Answer from the drawing. Dimensions are ordinates in mm from the lowest x, y and z of the part. A direction names the side the tool comes from. Round coordinates to 2 decimals unless told otherwise and drop trailing zeros. Loops run counter-clockwise (first coordinate to the right, second up) from the corner with the lowest first, then second, coordinate; pieces in that order, holes last. Notation, with made-up numbers: M 0,53 L 34,53 A23 ccw 34,70 Z; hole C 41.25,-29.5 d8. An arc over 180 degrees is marked long. Answer as CSV lines item,"result".
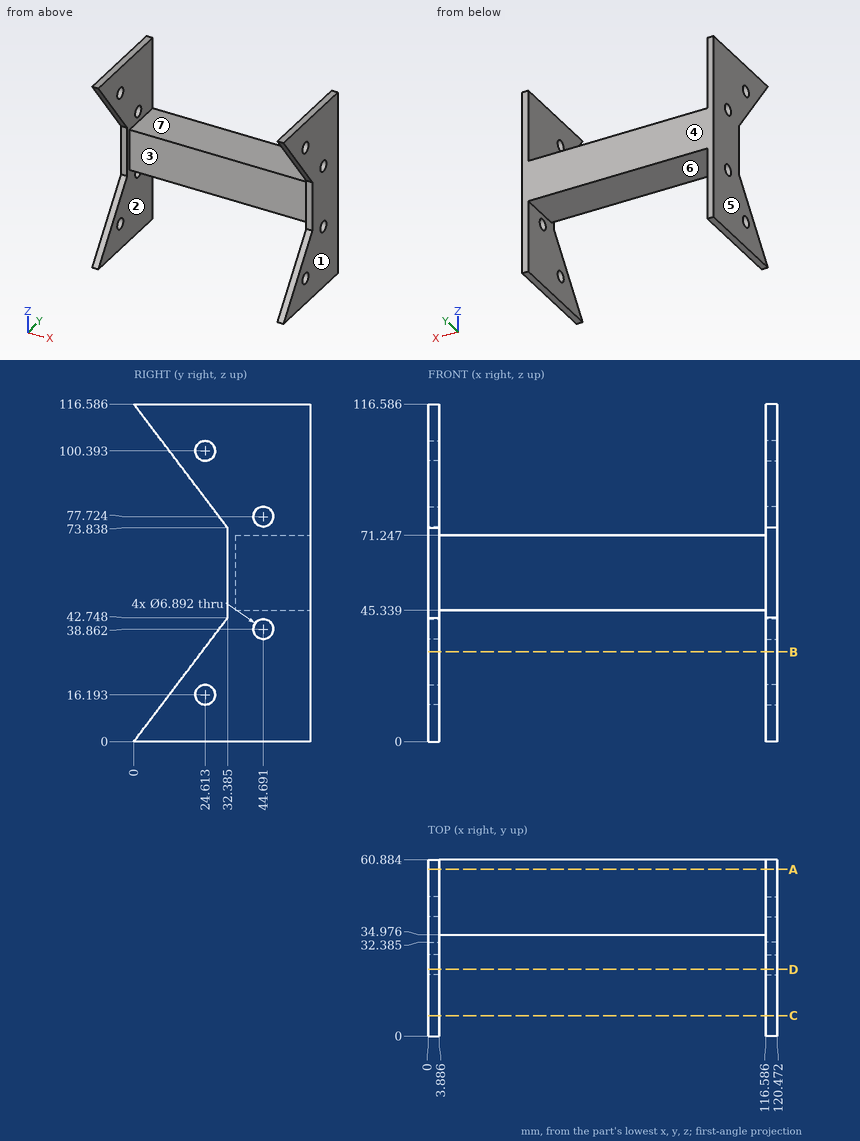
1) Find section D-D, the plane y = 23. Count the separate pieces of the cut face and the enclosed holes in it.
Evaluation:
separate pieces,"8"
enclosed holes,"0"
2) Find section A-A, the plane y = 57.5. Give the vertices of the cut face in (x, z) (1 decimal), then the cut area to 3 significant figures.
Evaluation:
outline,"M 0,0 L 3.9,0 L 3.9,45.3 L 116.6,45.3 L 116.6,0 L 120.5,0 L 120.5,116.6 L 116.6,116.6 L 116.6,71.2 L 3.9,71.2 L 3.9,116.6 L 0,116.6 Z"
area,"3,830 mm^2"
3) A tool of negligible diameter and unlimited length cuts with its end or side. For the marked faces 5, 6 and 7, from which of +Z, -Z, +X, -X, +Y, -Y can it reach the whole face along a straight path? Write none if from no direction.
Evaluation:
face 5,"+Z, -Z, -X, +Y, -Y"
face 6,"-Z, +Y, -Y"
face 7,"+Z, +Y, -Y"
4) Find section B-B, the plane z = 31. Give the vertices of the cut face in (x, y) (1 decimal).
Evaluation:
outline,"M 0,23.5 L 3.9,23.5 L 3.9,60.9 L 0,60.9 Z; M 116.6,23.5 L 120.5,23.5 L 120.5,60.9 L 116.6,60.9 Z"
5) Find section C-C, the plane y = 7. Give the vertices of the cut face in (x, z) (1 decimal), then the cut area to 3 significant figures.
Evaluation:
outline,"M 0,0 L 3.9,0 L 3.9,9.2 L 0,9.2 Z; M 0,107.3 L 3.9,107.3 L 3.9,116.6 L 0,116.6 Z; M 116.6,0 L 120.5,0 L 120.5,9.2 L 116.6,9.2 Z; M 116.6,107.3 L 120.5,107.3 L 120.5,116.6 L 116.6,116.6 Z"
area,"144 mm^2"
6) Each of these flat-tipped pins is pushed along its axis until it touches: P1, Ø6, axis at x = 40.5, z = 63, coming from the -Y side; P2, Ø1.9, axis at x = 3, z = 51.5, coming from the -Y side (1 decimal); P3, Ø6, axis at y = 44.69, z = 77.72, coming from the -X side; P4, Ø1.5, axis at x = 22, y = 38.5, coming from the -Z side. Where does it stop, or does it pass through?
Evaluation:
P1,"stops at y = 34.98"
P2,"stops at y = 32.4"
P3,"passes through"
P4,"stops at z = 45.34"
7) Determine the mould class of the marked faces 1, 2, 3 and 4 for opening direction X: released by +X, released by -X, zero draft, split by the parting line, or undercut.
Evaluation:
face 1,"released by +X"
face 2,"undercut"
face 3,"undercut"
face 4,"zero draft"
8) Straight lines are drawn through the part: line 1 (X direction, y = 35.5, z = 42) (1 decimal); line 2 (Z direction, x = 52.5, y = 46); line 3 (Y direction, x = 26, z = 52) (1 decimal). For each, find the intervals that lie inside material, in ascending order.
Evaluation:
line 1,"x = 0 to 3.9, 116.6 to 120.5"
line 2,"z = 45.34 to 71.25"
line 3,"y = 35 to 60.9"
